Autodesk Inventor part; units mm, degrees
ref_plane "YZ Plane" through (0, 0, 0) normal (1, 0, 0) x (0, 1, 0)
ref_plane "XZ Plane" through (0, 0, 0) normal (0, 1, 0) x (-1, 0, 0)
ref_plane "XY Plane" through (0, 0, 0) normal (0, 0, 1) x (1, 0, 0)
sketch "Sketch1" plane through (0, 0, 0) normal (0, 0, 1) x (1, 0, 0)
  line L0 (-136.525, 38.1) -> (136.525, 38.1)
  line L1 (136.525, 38.1) -> (136.525, -38.1)
  line L2 (136.525, -38.1) -> (-136.525, -38.1)
  line L3 (-136.525, -38.1) -> (-136.525, 38.1)
  line L4 (0, 0) -> (0, 38.1) construction
  line L5 (0, 0) -> (0, -38.1) construction
  line L6 (0, 0) -> (-136.525, 0) construction
  line L7 (0, 0) -> (136.525, 0) construction
  dimension "d0" = 273.05
  dimension "d1" = 76.2
extrude "PCB" add sketch "Sketch1" along normal mid plane 2.2098
sketch "Sketch2" plane through (0, 0, 1.1049) normal (0, 0, 1) x (1, 0, 0)
  line L0 (-136.525, 38.1) -> (136.525, 38.1)
  line L1 (-136.525, -38.1) -> (-136.525, 38.1)
  line L2 (136.525, -38.1) -> (-136.525, -38.1)
  line L3 (-122.5042, 33.9217) -> (-122.5042, 38.1) construction
  line L4 (-122.5042, -33.9217) -> (-122.5042, -38.1) construction
  point P0 (-29.4894, 33.9217)
  point P1 (18.0848, 33.9217)
  point P2 (112.5728, 33.9217)
  point P3 (-40.9702, -33.9217)
  point P4 (18.0848, -33.9217)
  point P5 (112.5728, -33.9217)
  dimension "d4" = 67.8434
  dimension "d5" = 14.0208
  dimension "d6" = 93.0148
  dimension "d7" = 47.5742
  dimension "d8" = 94.488
  dimension "d9" = 81.534
hole "Hole1" at (-122.5042, 33.9217, 1.1049) at (-122.5042, -33.9217, 1.1049) at (-29.4894, 33.9217, 1.1049) at (18.0848, 33.9217, 1.1049) at (112.5728, 33.9217, 1.1049) at (-40.9702, -33.9217, 1.1049) at (18.0848, -33.9217, 1.1049) at (112.5728, -33.9217, 1.1049) direction (0, 0, -1) diameter 3.429 end through all
sketch "Sketch3" plane through (0, 0, 1.1049) normal (0, 0, 1) x (1, 0, 0)
  circle A0 centre (18.0848, -33.9217) radius 1.7145
  circle A1 centre (-40.9702, -33.9217) radius 1.7145
  point P0 (-40.9702, -7.6581)
  point P1 (124.1298, -7.6581)
  dimension "d17" = 165.1
  dimension "d18" = 26.2636
  dimension "d19" = 59.055
hole "Hole2" at (-40.9702, -7.6581, 1.1049) at (124.1298, -7.6581, 1.1049) direction (0, 0, -1) diameter 11.0744 end through all
properties part number "cRIO Electric Board 1764" material "Phenolic"
The listing builds one solid part. Answer for the finished solid, in the listing's coordinates (mm). Round coordinates to 2 decimals unless told otherwise and drop trailing zeros. Write each loop counter-clockwise with the first axis right and the second up, starting at its lowest first coordinate (ties: lowest second). Pieces come first, ordered by that corner, then holes. Notation, with made-up numbers: (52.25, 67.5) -> (89.25, 67.5) arc R31 ccw to (89.25, 100.5) -> close; hole circle Ø10 at (49, 51). An arc over 180 degrees is marked (long way). Answer as a JSON object with one key per item and string values. Group by question number.
Q1. This flat-tipped pin is pushed along its axis until it touches: pin 1 Ø4.5 at (x, y) = (18.08, 33.92) entering from +Z. Where does it stop, or does it pass through?
Q2. Section A-A (y = -8) is taken. Write down the section's boundary in (x, z) (3 decimals).
Q3. Straight lines are drawn through the part: line 1 along X through (y, z) = (-7.5, 0.75) (3 decimals); line 2 along X through (y, z) = (-3, 0.7) (3 decimals); line 3 along X through (y, z) = (33, 0.5) (3 decimals). For each, find the intervals that lie inside material, in ascending order.
Q4. Determine the mould class of faces 1 (the face through (-2, 1, 1.105)), 2 (the face through (-46.46, -6.94, -0.02)) for opening direction Y: pulls with the +Y half, pulls with the -Y half, needs draft (parallel to the pull), parting line crosses it, or undercut.
Check values:
{
 "1": {"pin 1": "z = 1.1"},
 "2": {"outline": "(-136.525, -1.105) -> (-46.497, -1.105) -> (-46.497, 1.105) -> (-136.525, 1.105) -> close; (-35.444, -1.105) -> (118.603, -1.105) -> (118.603, 1.105) -> (-35.444, 1.105) -> close; (129.656, -1.105) -> (136.525, -1.105) -> (136.525, 1.105) -> (129.656, 1.105) -> close"},
 "3": {"line 1": "-136.525 to -46.505, -35.435 to 118.595, 129.665 to 136.525", "line 2": "-136.525 to -43.964, -37.976 to 121.136, 127.124 to 136.525", "line 3": "-136.525 to -123.95, -121.059 to -30.935, -28.044 to 16.639, 19.53 to 111.127, 114.018 to 136.525"},
 "4": {"face 1": "needs draft", "face 2": "undercut"}
}
